Geometry: final body of the model. Coordinates: model frame, mm. A direction names the side the tool comes from. Round coordinates to 2 decimals unless told otherwise and drop trailing zeros. Write each loop counter-clockwise with the first axis right and the second up, starting at its lowest first coordinate (ties: lowest second). Pieces come first, ordered by that corner, then holes. Notation, with made-up numbers: M 5.25,11 L 50.25,11 A16 ccw 50.25,22 Z; hole C -39,15.5 d2. An arc over 180 degrees is marked long. Use one line per item in the form item = value. Start each with the question number.
Item 1: Ray query, probe 1 along X at (y, z) = (1.75, -3.5); probe 2 along Z at (x, y) = (-13.5, 2.5); probe 3 along Y at (x, z) = (42, 24.5). Return the intervals inside material, ascending.
Item 2: Section query B-B (z = 26). Return loops of the section in (x, y), and give its area (3 significant figures).
Item 3: Section query C-C (x = -4.5). Return loops of the section in (y, z), and give its area (3 significant figures).
Item 4: Reachability of faces 1 (the flat face through (23, 3, 29.265)), 2 (the flat face through (75.7, 3, 8)), 3 (the flat face through (25, 3, -13.375)), 4 (the flat face through (23, 0, 8)), 5 (the flat face through (25, 3, 28.265)) from +Z, -Z, +X, -X, +Y, -Y: full face, straight path, thin tool, end or side. Return the list, or none.
Item 5: Section query A-A (y = 4.5). Return loops of the section in (x, z).
Item 6: Pull-direction query (X, two-part tool) for faces 6 (the flat face through (24, 1.6, -14)), 7 (the flat face through (-27.9, 3, 8)), 8 (the flat face through (74.7, 3, 8)), 9 (the flat face through (23, 1.6, 8)); classes: pulls with the +X half, pulls with the -X half, needs draft (parallel to the pull), parting line crosses it, or undercut.
Item 7: Pin query (flat end, axial travel): pin 1 Ø8 at (x, z) = (43.5, 11) entering from +Y; pin 2 Ø0.8 at (x, y) = (-27.5, 4.5) entering from -Z; pin 3 Ø1.6 at (y, z) = (4, 0.5) entering from +X; pin 4 Ø2 at (x, y) = (17, 2) entering from +Z. Return the tip coordinate at first contact, or that it passes through.
from build123d import *

# Parameters (mm, degrees)
SKETCH1_W           = 105.6
SKETCH1_H           = 44.64
SKETCH1_W_2         = 103.6
SKETCH1_H_2         = 42.64
SKETCH1_W_3         = 1
SKETCH1_H_3         = 4.4
SKETCH1_W_4         = 101.6
SKETCH1_H_4         = 40.64
BOSS_EXTRUDE1_DEPTH = 1.6
SKETCH1_3_W         = 1
SKETCH1_3_H         = 4.4
BOSS_EXTRUDE2_DEPTH = 3.45
SKETCH1_4_W         = 1
SKETCH1_4_H         = 4.4
BOSS_EXTRUDE3_DEPTH = 6.8


with BuildPart() as part:
    # Sketch1 → Boss-Extrude1 (new body)
    # profile 1 of 6: a face of its own
    with BuildSketch(Plane(origin=(0, 0, 0), x_dir=(1, 0, 0), z_dir=(0, 1, 0))):
        with Locations((23.9, -7.945434783)):
            Rectangle(SKETCH1_W, SKETCH1_H)
        with Locations((23.9, -7.945434783)):
            Rectangle(SKETCH1_W_2, SKETCH1_H_2, mode=Mode.SUBTRACT)
    # profile 2 of 6: a face of its own
    with BuildSketch(Plane(origin=(0, 0, 0), x_dir=(1, 0, 0), z_dir=(0, 1, 0))):
        Polygon((-26.9, -10.145434783), (-27.9, -10.145434783), (-27.9, -29.265434783), (75.7, -29.265434783), (75.7, -10.145434783), (74.7, -10.145434783), (74.7, -28.265434783), (-26.9, -28.265434783), align=None)
    # profile 3 of 6: a face of its own
    with BuildSketch(Plane(origin=(0, 0, 0), x_dir=(1, 0, 0), z_dir=(0, 1, 0))):
        with Locations((-27.4, -7.945434783)):
            Rectangle(SKETCH1_W_3, SKETCH1_H_3)
    # profile 4 of 6: a face of its own
    with BuildSketch(Plane(origin=(0, 0, 0), x_dir=(1, 0, 0), z_dir=(0, 1, 0))):
        Polygon((75.7, 13.374565217), (-27.9, 13.374565217), (-27.9, -5.745434783), (-26.9, -5.745434783), (-26.9, 12.374565217), (74.7, 12.374565217), (74.7, -5.745434783), (75.7, -5.745434783), align=None)
    # profile 5 of 6: a face of its own
    with BuildSketch(Plane(origin=(0, 0, 0), x_dir=(1, 0, 0), z_dir=(0, 1, 0))):
        with Locations((23.9, -7.945434783)):
            Rectangle(SKETCH1_W_4, SKETCH1_H_4)
    # profile 6 of 6: a face of its own
    with BuildSketch(Plane(origin=(0, 0, 0), x_dir=(1, 0, 0), z_dir=(0, 1, 0))):
        with Locations((75.2, -7.945434783)):
            Rectangle(SKETCH1_W_3, SKETCH1_H_3)
    extrude(amount=BOSS_EXTRUDE1_DEPTH)

    # Sketch1_3 → Boss-Extrude2 (add)
    with BuildSketch(Plane(origin=(0, 0, 0), x_dir=(1, 0, 0), z_dir=(0, 1, 0))):
        Polygon((75.7, 13.374565217), (-27.9, 13.374565217), (-27.9, -5.745434783), (-26.9, -5.745434783), (-26.9, 12.374565217), (74.7, 12.374565217), (74.7, -5.745434783), (75.7, -5.745434783), align=None)
        Polygon((-26.9, -10.145434783), (-27.9, -10.145434783), (-27.9, -29.265434783), (75.7, -29.265434783), (75.7, -10.145434783), (74.7, -10.145434783), (74.7, -28.265434783), (-26.9, -28.265434783), align=None)
        with Locations((-27.4, -7.945434783)):
            Rectangle(SKETCH1_3_W, SKETCH1_3_H)
        with Locations((75.2, -7.945434783)):
            Rectangle(SKETCH1_3_W, SKETCH1_3_H)
    extrude(amount=BOSS_EXTRUDE2_DEPTH)

    # Sketch1_4 → Boss-Extrude3 (add)
    with BuildSketch(Plane(origin=(0, 0, 0), x_dir=(1, 0, 0), z_dir=(0, 1, 0))):
        with Locations((75.2, -7.945434783)):
            Rectangle(SKETCH1_4_W, SKETCH1_4_H)
        with Locations((-27.4, -7.945434783)):
            Rectangle(SKETCH1_4_W, SKETCH1_4_H)
    extrude(amount=BOSS_EXTRUDE3_DEPTH)


solid = part.part
Working result:
q1.probe_1 = -27.9 to -26.9, 74.7 to 75.7
q1.probe_2 = -13.37 to -12.37, 28.27 to 29.27
q1.probe_3 = 0 to 1.6
q2.outline = M -28.9,0 L 76.7,0 L 76.7,1.6 L 75.7,1.6 L 75.7,3.45 L 74.7,3.45 L 74.7,1.6 L -26.9,1.6 L -26.9,3.45 L -27.9,3.45 L -27.9,1.6 L -28.9,1.6 Z
q2.area = 173 mm²
q3.outline = M 0,-14.37 L 1.6,-14.37 L 1.6,-13.37 L 3.45,-13.37 L 3.45,-12.37 L 1.6,-12.37 L 1.6,28.27 L 3.45,28.27 L 3.45,29.27 L 1.6,29.27 L 1.6,30.27 L 0,30.27 Z
q3.area = 75.1 mm²
q4.face_1 = +Z, +X, -X, +Y
q4.face_2 = +Z, -Z, +X, +Y
q4.face_3 = -Z, +X, -X, +Y
q4.face_4 = +Z, -Z, +X, -X, -Y
q4.face_5 = +Y
q5.outline = M -27.9,5.75 L -26.9,5.75 L -26.9,10.15 L -27.9,10.15 Z; M 74.7,5.75 L 75.7,5.75 L 75.7,10.15 L 74.7,10.15 Z
q6.face_6 = needs draft
q6.face_7 = pulls with the -X half
q6.face_8 = undercut
q6.face_9 = undercut
q7.pin_1 = 1.6
q7.pin_2 = 5.75
q7.pin_3 = 75.7
q7.pin_4 = 30.27
